Check sheet for the modelled part. Datum: model origin and axes. Units: mm. A direction names the side the tool comes from. Round coordinates to 2 decimals unless told otherwise and drop trailing zeros. Write each loop counter-clockwise with the first axis right and the second up, starting at its lowest first coordinate (ties: lowest second). Pieces come first, ordered by that corner, then holes. Notation, with made-up numbers: M 68.5,25.5 L 91.5,25.5 A35 ccw 91.5,63.5 Z; hole C 89,15.5 d10. An arc over 180 degrees is marked long. Answer in a Markdown table with one row per item.
```python
from build123d import *

# Parameters (mm, degrees)
SKETCH2_W           = 57
SKETCH2_H           = 57
BOSS_EXTRUDE1_DEPTH = 35
SKETCH3_W           = 5
SKETCH3_H           = 1
CUT_EXTRUDE1_DEPTH  = 60
SKETCH4_W           = 49.5
SKETCH4_H           = 49.5
CUT_EXTRUDE2_DEPTH  = 28
CUT_EXTRUDE4_DEPTH  = 5
CUT_EXTRUDE5_DEPTH  = 10
SKETCH13_W          = 7
SKETCH13_H          = 1.952566844
CUT_EXTRUDE8_DEPTH  = 12


with BuildPart() as part:
    # Sketch2 → Boss-Extrude1 (new body)
    with BuildSketch(Plane.XY):
        with Locations((-5.733009709, -0.737864078)):
            Rectangle(SKETCH2_W, SKETCH2_H)
    extrude(amount=BOSS_EXTRUDE1_DEPTH)

    # Sketch3 → Cut-Extrude1 (cut)
    with BuildSketch(Plane(origin=(0, 27.762135922, 0), x_dir=(1, 0, 0), z_dir=(0, 1, 0))):
        with Locations((-27.733009709, -32.5)):
            Rectangle(SKETCH3_W, SKETCH3_H)
        with Locations((16.266990291, -32.5)):
            Rectangle(SKETCH3_W, SKETCH3_H)
    extrude(amount=-CUT_EXTRUDE1_DEPTH, mode=Mode.SUBTRACT)

    # Sketch4 → Cut-Extrude2 (cut)
    with BuildSketch(Plane(origin=(0, 0, 0), x_dir=(-1, 0, 0), z_dir=(0, 0, -1))):
        with Locations((5.733009709, -0.737864078)):
            Rectangle(SKETCH4_W, SKETCH4_H)
    extrude(amount=-CUT_EXTRUDE2_DEPTH, mode=Mode.SUBTRACT)

    # Sketch5 → Cut-Extrude4 (cut)
    with BuildSketch(Plane(origin=(0, -25.487864078, 0), x_dir=(1, 0, 0), z_dir=(0, 1, 0))):
        with BuildLine():
            Line((2.766990291, -12), (2.766990291, 0))
            Line((2.766990291, 0), (-14.233009709, 0))
            Line((-14.233009709, 0), (-14.233009709, -12))
            ThreePointArc((-14.233009709, -12), (-5.733009709, -20.5), (2.766990291, -12))
        make_face()
    extrude(amount=-CUT_EXTRUDE4_DEPTH, mode=Mode.SUBTRACT)

    # Sketch7 → Cut-Extrude5 (cut)
    with BuildSketch(Plane(origin=(-30.483009709, 0, 0), x_dir=(0, 0, -1), z_dir=(1, 0, 0))):
        with BuildLine():
            Line((-12, -9.237864078), (0, -9.237864078))
            Line((0, -9.237864078), (0, 7.762135922))
            Line((0, 7.762135922), (-12, 7.762135922))
            ThreePointArc((-12, 7.762135922), (-20.5, -0.737864078), (-12, -9.237864078))
        make_face()
    extrude(amount=-CUT_EXTRUDE5_DEPTH, mode=Mode.SUBTRACT)

    # Sketch13 → Cut-Extrude8 (cut)
    with BuildSketch(Plane(origin=(0, 27.762135922, 0), x_dir=(1, 0, 0), z_dir=(0, 1, 0))):
        with Locations((8.266990291, -4.976283422)):
            Rectangle(SKETCH13_W, SKETCH13_H)
    extrude(amount=-CUT_EXTRUDE8_DEPTH, mode=Mode.SUBTRACT)


solid = part.part
```
1. Scan lines: L1, parallel to X at y = 9, z = 25; L2, parallel to Z at x = -26, y = -16; L3, parallel to X at y = 17.5, z = 32.5. Record each from-to range of solid material in increasing order.
Found:
| item | result |
|---|---|
| L1 | x = -34.23 to -30.48, 19.02 to 22.77 |
| L2 | z = 28 to 32, 33 to 35 |
| L3 | x = -34.23 to -30.23, -25.23 to 13.77, 18.77 to 22.77 |
2. Section check B-B, the plane y = 22. Record the cut outline in (x, z), and give its area (3 significant figures).
Found:
| item | result |
|---|---|
| outline | M -34.23,0 L -30.48,0 L -30.48,28 L 19.02,28 L 19.02,0 L 22.77,0 L 22.77,35 L -34.23,35 Z; hole M -30.23,32 L -25.23,32 L -25.23,33 L -30.23,33 Z; hole M 13.77,32 L 18.77,32 L 18.77,33 L 13.77,33 Z |
| area | 599 mm2 |
3. Section check A-A, the plane z = 7.5. Record the cut outline in (x, y).
Found:
| item | result |
|---|---|
| outline | M -34.23,-29.24 L -14.23,-29.24 L -14.23,-25.49 L -30.48,-25.49 L -30.48,-9.24 L -34.23,-9.24 Z; M -34.23,7.76 L -30.48,7.76 L -30.48,24.01 L 19.02,24.01 L 19.02,-25.49 L 2.77,-25.49 L 2.77,-29.24 L 22.77,-29.24 L 22.77,27.76 L -34.23,27.76 Z |
4. Draft check along Y on faces 1 (the face through (11.767, 26, 5)), 2 (the face through (-6, 27.762, 17)), 3 (the face through (-32.3, -0.6, 20.5)). Enter one of: +Y half, -Y half, draft (parallel to the pull), parting line (faces both ways), or undercut.
Found:
| item | result |
|---|---|
| face 1 | draft |
| face 2 | +Y half |
| face 3 | undercut |
5. Access from +Z, -Z, +X, -X, +Y, -Y to the whole of each face (thin tool, end or side, straight path). Record for faces 4 (the face through (22.767, -1, 17)), 5 (the face through (0, -25.488, 20)), 6 (the face through (3, 25, 0)), 7 (the face through (4.767, 26, 5)), 8 (the face through (-28, 0, 32)).
Found:
| item | result |
|---|---|
| face 4 | +Z, -Z, +X, +Y, -Y |
| face 5 | -Z |
| face 6 | -Z, +X, -X, +Y, -Y |
| face 7 | +Y |
| face 8 | +Y, -Y |
6. Section check D-D, the plane x = 1. Record the cut outline in (y, z).
Found:
| item | result |
|---|---|
| outline | M -29.24,17.19 L -25.49,17.19 L -25.49,28 L 24.01,28 L 24.01,0 L 27.76,0 L 27.76,35 L -29.24,35 Z |
7. Section check C-C, the plane z = 23.5. Record the cut outline in (x, y), and give its area (3 significant figures).
Found:
| item | result |
|---|---|
| outline | M -34.23,-29.24 L 22.77,-29.24 L 22.77,27.76 L -34.23,27.76 Z; hole M -30.48,-25.49 L 19.02,-25.49 L 19.02,24.01 L -30.48,24.01 Z |
| area | 799 mm2 |
8. Go/stop test with flat-tipped pins: pin 1 (2.5 mm diameter, centred on x = 16.5, y = -8.5, fed in from -Z); pin 2 (8.5 mm diameter, centred on y = 1, z = 9.5, fed in from -X). Record where each tip stops, or that it passes through.
Found:
| item | result |
|---|---|
| pin 1 | stops at z = 28 |
| pin 2 | stops at x = 19.02 |
